Part model, mm, in its own coordinate system. Face numbers are marked on the shaded views. A direction names the side the tool comes from. Give positions to 0.01 mm unless a question says otherwise; leave off trailing zeros. Order: outer loops, then holes, each group sorted by start corner. A loop starts at its lowest first (then second) coordinate and runs counter-clockwise, first axis right, second up.
1. Slice it at A-A on x = 0. List the corners of the cut face in (y, z) (3 decimals), and give its area (3 significant figures).
2. Probe line 1 (Y direction, x = 0, z = 2.05); line 2 (Y direction, x = 2.5, z = -0.25) (3 decimals); line 3 (Z direction, x = 6, y = -2.75) (3 decimals). List the from-to ranges inside material, lowest first.
3. Slice it at C-C on z = -1.75. List the corners of the cut face in (x, y) (3 decimals).
4. Which spindle directions (+Z, -Z, +X, -X, +Y, -Y) get a long thin tool onto all of the face, cutting with end or side? Do the marked faces 1 and 2. Say none if no direction does.
5. Drop flat-ended pins along their axis: pin 1 Ø1.9 at (x, z) = (3.5, -4) entering from -Y; pin 2 Ø4 at (x, z) = (-6.5, -6) entering from +Y; pin 3 Ø4 at (x, z) = (-10, -6) entering from -Y. Give the stop position or say it passes through.
6. Mould opens along Y. For the marked faces 3, 4, 5 and 6 say: +Y half, -Y half, draft (parallel to the pull), parting line (faces both ways), or undercut.
7. Slice it at D-D on z = 1.5. List the corners of the cut face in (x, y).
8. Slice it at B-B on y = 0. List the corners of the cut face in (x, z) (3 decimals), and give its area (3 significant figures).
from build123d import *

# Parameters (mm, degrees)
SKETCH1_R           = 14
BOSS_EXTRUDE1_DEPTH = 3.175
BOSS_EXTRUDE2_START = 12.7
BOSS_EXTRUDE2_DEPTH = 12.7
SKETCH3_W           = 6.35
SKETCH3_H           = 6.35
CUT_EXTRUDE1_DEPTH  = 38.333803689
SKETCH4_R           = 1.5
CUT_EXTRUDE2_DEPTH  = 27.995101119


with BuildPart() as part:
    # Sketch1 → Boss-Extrude1 (new body)
    with BuildSketch(Plane.XY):
        Circle(SKETCH1_R)
    extrude(amount=BOSS_EXTRUDE1_DEPTH)

    # Sketch2 → Boss-Extrude2 (add)
    with BuildSketch(Plane(origin=(0, 0, 3.175), x_dir=(-1, 0, 0), z_dir=(0, 0, -1)).offset(BOSS_EXTRUDE2_START)):
        with BuildLine():
            Line((-12.477078985, 6.35), (19.272921015, 6.35))
            Line((19.272921015, 6.35), (19.272921015, -6.35))
            Line((19.272921015, -6.35), (-12.477078985, -6.35))
            ThreePointArc((-12.477078985, -6.35), (-14, 0), (-12.477078985, 6.35))
        make_face()
    extrude(amount=-BOSS_EXTRUDE2_DEPTH)

    # Sketch3 → Cut-Extrude1 (cut, through all)
    with BuildSketch(Plane.ZY.offset(19.272921015)):
        with Locations((-3.175, 0)):
            Rectangle(SKETCH3_W, SKETCH3_H)
    extrude(amount=-CUT_EXTRUDE1_DEPTH, mode=Mode.SUBTRACT)

    # Sketch4 → Cut-Extrude2 (cut, through all)
    with BuildSketch(Plane.XY.offset(3.175)):
        with Locations((-9.5, 0)):
            Circle(SKETCH4_R)
        with Locations(Location((9.5, 0, 0), (0, 0, 180))):
            Circle(SKETCH4_R)
        with Locations((0, 8)):
            Circle(SKETCH4_R)
        with Locations((0, -8)):
            Circle(SKETCH4_R)
    extrude(amount=-CUT_EXTRUDE2_DEPTH, mode=Mode.SUBTRACT)


solid = part.part
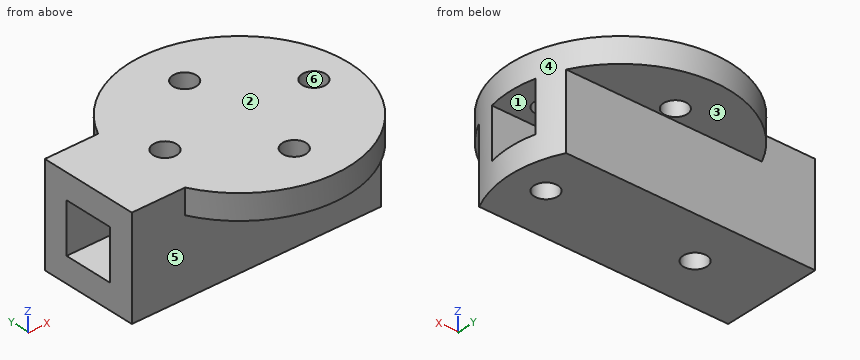
Data:
1. outline: (-14, 0) - (-9.5, 0) - (-9.5, 3.175) - (-14, 3.175) - close; (-6.5, 0) - (-6.35, 0) - (-6.35, -9.525) - (6.35, -9.525) - (6.35, 0) - (6.5, 0) - (6.5, 3.175) - (-6.5, 3.175) - close; (9.5, 0) - (14, 0) - (14, 3.175) - (9.5, 3.175) - close; hole (-3.175, -6.35) - (3.175, -6.35) - (3.175, 0) - (-3.175, 0) - close
1. area: 150 mm2
2. line 1: y = -14 to -9.5, -6.5 to 6.5, 9.5 to 14
2. line 2: y = -6.35 to -3.175, 3.175 to 6.35
2. line 3: z = -9.525 to -6.35, 0 to 3.175
3. outline: (-19.273, -6.35) - (12.477, -6.35) arc R14 ccw to (13.635, -3.175) - (-19.273, -3.175) - close; (-19.273, 3.175) - (13.635, 3.175) arc R14 ccw to (12.477, 6.35) - (-19.273, 6.35) - close
4. face 1: +X, -X
4. face 2: +Z, +X, -X, +Y, -Y
5. pin 1: stops at y = -6.35
5. pin 2: stops at y = 6.35
5. pin 3: stops at y = -6.35
6. face 3: draft
6. face 4: parting line
6. face 5: -Y half
6. face 6: undercut
7. outline: (-19.27, -6.35) - (-12.48, -6.35) arc R14 ccw (long way) to (-12.48, 6.35) - (-19.27, 6.35) - close; hole circle Ø3 at (-9.5, 0); hole circle Ø3 at (0, -8); hole circle Ø3 at (0, 8); hole circle Ø3 at (9.5, 0)
8. outline: (-19.273, -9.525) - (-11, -9.525) - (-11, -6.35) - (-19.273, -6.35) - close; (-19.273, 0) - (-11, 0) - (-11, 3.175) - (-19.273, 3.175) - close; (-8, -9.525) - (8, -9.525) - (8, -6.35) - (-8, -6.35) - close; (-8, 0) - (8, 0) - (8, 3.175) - (-8, 3.175) - close; (11, -9.525) - (14, -9.525) - (14, -6.35) - (11, -6.35) - close; (11, 0) - (14, 0) - (14, 3.175) - (11, 3.175) - close
8. area: 173 mm2
